The listing builds one solid part. Answer for the finished solid, in the listing's coordinates (mm). Face numbers are marked on the shaded views. A direction names the side the tool comes from. Give positions to 0.01 mm unless a question says otherwise; leave off trailing zeros. Order: outer loops, then holes, each group sorted by start corner. A loop starts at its lowest first (then second) coordinate and runs counter-clockwise, first axis right, second up. Notation, with made-up numbers: (81, 52) - (99, 52) arc R27 ccw to (99, 83) - close; hole circle Ø3 at (45.25, -9). An arc over 180 degrees is marked (long way). Write each question's results on one line, items separated by ' | '. Start each with the question number.
1. Which of the six approach directions +Z, -Z, +X, -X, +Y, -Y give full straight-line access (tool end or side, diameter ignored) to the marked faces 1 and 2?
2. Find the intervals of material crossed by L1, parallel to Y at x = 18.5, z = 19.5; L2, parallel to X at y = 91.5, z = -22; L3, parallel to Z at x = -9.5, y = 45, in increasing order.
3. Section A-A (z = 0) is taken. Give the vertices of the cut face in (x, y), and give its area (3 significant figures).
4. Flat-ended cylindrical pins translate along their axes: pin 1 (3 mm diameter, centred on x = 7, y = 21, fed in from +Z); pin 2 (2 mm diameter, centred on x = -4, y = 72, fed in from +Z); pin 3 (3 mm diameter, centred on x = -25.5, z = 22, fed in from +Y). Find the tip coordinate at first contact, or state that the pin passes through.
from build123d import *

# Parameters (mm, degrees)
SKIZZE1_R                       = 25
AUFSATZ_LINEAR_AUSTRAGEN1_DEPTH = 100
SKIZZE2_R                       = 32.5
AUFSATZ_LINEAR_AUSTRAGEN2_DEPTH = 20
FORMSCHR_GE1_ANGLE              = 2
VERRUNDUNG1_R                   = 2


with BuildPart() as part:
    # Skizze1 → Aufsatz-Linear austragen1 (new body)
    with BuildSketch(Plane(origin=(0, 0, 0), x_dir=(1, 0, 0), z_dir=(0, 1, 0))):
        with Locations(Location((0, 0, 0), (0, 0, 270))):  # turned: the seam where the file's is
            Circle(SKIZZE1_R)
    extrude(amount=AUFSATZ_LINEAR_AUSTRAGEN1_DEPTH)

    # Skizze2 → Aufsatz-Linear austragen2 (add)
    with BuildSketch(Plane.XZ):
        with Locations(Location((0, 0, 0), (0, 0, 270))):  # turned: the seam where the file's is
            Circle(SKIZZE2_R)
    extrude(amount=AUFSATZ_LINEAR_AUSTRAGEN2_DEPTH)

    # Formschräge1
    formschr_ge1_faces = [part.faces().sort_by_distance(p)[0] for p in [
        (0, 50, -25),
    ]]
    draft(formschr_ge1_faces, Plane.ZX, FORMSCHR_GE1_ANGLE)

    # Austragung6: sweep along a path in Skizze6
    with BuildLine(Plane(origin=(0, 0, 0), x_dir=(0, 0, -1), z_dir=(1, 0, 0))) as austragung6_path:
        Line((21.507923051, 100), (25, 0))
    # Skizze8 → Austragung6 (sweep)
    with BuildSketch(Plane(origin=(0, 100, 0), x_dir=(1, 0, 0), z_dir=(0, 1, 0))):
        with BuildLine():
            ThreePointArc((4.290296742, 21.075675738), (0, 23.507923051), (-4.290296742, 21.075675738))
            ThreePointArc((-4.290296742, 21.075675738), (0, 21.507923051), (4.290296742, 21.075675738))
        make_face()
    sweep(path=austragung6_path.line)

    # Verrundung1
    verrundung1_edges = [part.edges().sort_by_distance(p)[0] for p in [
        (-4.267773944, 50.000105853, -22.858973285),
        (4.267773944, 50.000105853, -22.858973285),
    ]]
    fillet(verrundung1_edges, radius=VERRUNDUNG1_R)


solid = part.part
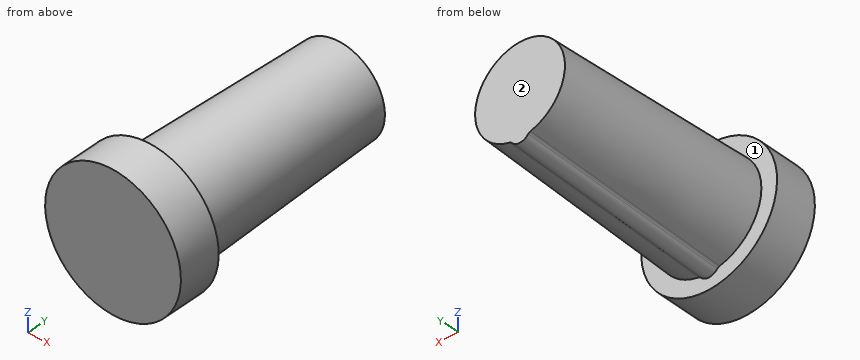
Reported:
1) face 1: +Y | face 2: +Z, -Z, +X, -X, +Y
2) L1: -20 to 0 | L2: -3.85 to 3.85 | L3: -21.42 to 21.42
3) outline: (-32.5, -20) - (32.5, -20) - (32.5, 0) - (25, 0) - (21.51, 100) - (-21.51, 100) - (-25, 0) - (-32.5, 0) - close | area: 5,950 mm²
4) pin 1: z = 23.64 | pin 2: z = 22.29 | pin 3: y = 0
